from build123d import *

# Parameters (mm, degrees)
SKETCH1_W               = 2.3
SKETCH1_H               = 5.5
SKETCH1_R               = 2.25
BOSS_EXTRUDE1_DEPTH     = 15
CUT_EXTRUDE1_DEPTH      = 33.128647653
CUT_EXTRUDE1_DEPTH_BACK = 33.128647653
SKETCH2_R               = 1.75
FILLET2_R               = 1.5
SKETCH4_R               = 5
CUT_EXTRUDE2_DEPTH      = 10


with BuildPart() as part:
    # Sketch1 → Boss-Extrude1 (new body)
    with BuildSketch(Plane(origin=(0, 0, 0), x_dir=(1, 0, 0), z_dir=(0, 1, 0))):
        with BuildLine():
            Line((15.13, 6.5), (-15.13, 6.5))
            ThreePointArc((-15.13, 6.5), (-18.573610024, 5.073610024), (-20, 1.63))
            Line((-20, 1.63), (-20, -1.63))
            ThreePointArc((-20, -1.63), (-18.573610024, -5.073610024), (-15.13, -6.5))
            Line((-15.13, -6.5), (-6.5, -6.5))
            ThreePointArc((-6.5, -6.5), (-5.439339828, -6.939339828), (-5, -8))
            Line((-5, -8), (-5, -12))
            ThreePointArc((-5, -12), (-4.560660172, -13.060660172), (-3.5, -13.5))
            Line((-3.5, -13.5), (-1, -13.5))
            Line((-1, -13.5), (-1, -3.97617907))
            ThreePointArc((-1, -3.97617907), (-2.520912533, 3.233419243), (4.1, 0))
            ThreePointArc((4.1, 0), (3.233419243, -2.520912533), (1, -3.97617907))
            Line((1, -3.97617907), (1, -13.5))
            Line((1, -13.5), (5.587465673, -13.5))
            Line((5.587465673, -13.5), (7.087465673, -13.5))
            ThreePointArc((7.087465673, -13.5), (8.148125845, -13.060660172), (8.587465673, -12))
            Line((8.587465673, -12), (8.587465673, -8))
            ThreePointArc((8.587465673, -8), (9.026805501, -6.939339828), (10.087465673, -6.5))
            Line((10.087465673, -6.5), (15.13, -6.5))
            ThreePointArc((15.13, -6.5), (18.573610024, -5.073610024), (20, -1.63))
            Line((20, -1.63), (20, 1.63))
            ThreePointArc((20, 1.63), (18.573610024, 5.073610024), (15.13, 6.5))
        make_face()
        with Locations((5, -10)):
            Rectangle(SKETCH1_W, SKETCH1_H, mode=Mode.SUBTRACT)
        with Locations(Location((-13, 0, 0), (0, 0, 270))):
            Circle(SKETCH1_R, mode=Mode.SUBTRACT)
        with Locations(Location((13, 0, 0), (0, 0, 270))):
            Circle(SKETCH1_R, mode=Mode.SUBTRACT)
    extrude(amount=BOSS_EXTRUDE1_DEPTH)

    # Sketch2 → Cut-Extrude1 (cut, two sides: drawn at the far end of the back side and taken through both)
    with BuildSketch(Plane(origin=(5, 0, 0), x_dir=(0, 0, -1), z_dir=(1, 0, 0)).offset(-CUT_EXTRUDE1_DEPTH_BACK)):
        with Locations((-10, 7.5)):
            Circle(SKETCH2_R)
    extrude(amount=CUT_EXTRUDE1_DEPTH + CUT_EXTRUDE1_DEPTH_BACK, mode=Mode.SUBTRACT)

    # Fillet2
    # the kernel refuses this fillet: 1.5 mm, written as the material it takes off along each edge
    with BuildSketch(Plane(origin=(7.087465673, 15, 13.5), x_dir=(0, 0, -1), z_dir=(-1, 0, 0))) as fillet2_piece_1:
        with BuildLine():
            CenterArc((FILLET2_R, FILLET2_R), FILLET2_R, 180, 90)
            Line((0, FILLET2_R), (0, 0))
            Line((0, 0), (FILLET2_R, 0))
        make_face()
    extrude(amount=9.837465673, mode=Mode.SUBTRACT)
    with BuildSketch(Plane(origin=(10.087465673, 15, 6.5), x_dir=(0, 0, -1), z_dir=(1, 0, 0))) as fillet2_piece_2:
        with BuildLine():
            CenterArc((FILLET2_R, -FILLET2_R), FILLET2_R, 90, 90)
            Line((0, -FILLET2_R), (0, 0))
            Line((0, 0), (FILLET2_R, 0))
        make_face()
    extrude(amount=5.042534327, mode=Mode.SUBTRACT)
    with BuildSketch(Plane(origin=(15.13, 15, 1.63), x_dir=(0, 0, 1), z_dir=(-1, 0, 0))) as fillet2_piece_3:
        with BuildLine():
            CenterArc((4.87 - FILLET2_R, -FILLET2_R), FILLET2_R, 0, 90)
            Line((4.87, -FILLET2_R), (4.87, 0))
            Line((4.87, 0), (4.87 - FILLET2_R, 0))
        make_face()
    revolve(axis=Axis((15.13, 15, 1.63), (0, 1, 0)), revolution_arc=90, mode=Mode.SUBTRACT)
    with BuildSketch(Plane(origin=(20, 15, 1.63), x_dir=(-1, 0, 0), z_dir=(0, 0, -1)), Plane(origin=(-20, 15, -1.63), x_dir=(1, 0, 0), z_dir=(0, 0, 1))) as fillet2_piece_4:
        with BuildLine():
            CenterArc((FILLET2_R, -FILLET2_R), FILLET2_R, 90, 90)
            Line((0, -FILLET2_R), (0, 0))
            Line((0, 0), (FILLET2_R, 0))
        make_face()
    extrude(amount=3.26, mode=Mode.SUBTRACT)
    with BuildSketch(Plane(origin=(15.13, 15, -1.63), x_dir=(1, 0, 0), z_dir=(0, 0, 1))) as fillet2_piece_5:
        with BuildLine():
            CenterArc((4.87 - FILLET2_R, -FILLET2_R), FILLET2_R, 0, 90)
            Line((4.87, -FILLET2_R), (4.87, 0))
            Line((4.87, 0), (4.87 - FILLET2_R, 0))
        make_face()
    revolve(axis=Axis((15.13, 15, -1.63), (0, 1, 0)), revolution_arc=90, mode=Mode.SUBTRACT)
    with BuildSketch(Plane(origin=(15.13, 15, -6.5), x_dir=(0, 0, 1), z_dir=(-1, 0, 0))) as fillet2_piece_6:
        with BuildLine():
            CenterArc((FILLET2_R, -FILLET2_R), FILLET2_R, 90, 90)
            Line((0, -FILLET2_R), (0, 0))
            Line((0, 0), (FILLET2_R, 0))
        make_face()
    extrude(amount=30.26, mode=Mode.SUBTRACT)
    with BuildSketch(Plane(origin=(-15.13, 15, -1.63), x_dir=(0, 0, -1), z_dir=(1, 0, 0))) as fillet2_piece_7:
        with BuildLine():
            CenterArc((4.87 - FILLET2_R, -FILLET2_R), FILLET2_R, 0, 90)
            Line((4.87, -FILLET2_R), (4.87, 0))
            Line((4.87, 0), (4.87 - FILLET2_R, 0))
        make_face()
    revolve(axis=Axis((-15.13, 15, -1.63), (0, 1, 0)), revolution_arc=90, mode=Mode.SUBTRACT)
    with BuildSketch(Plane(origin=(-3.5, 15, 13.5), x_dir=(0, 0, -1), z_dir=(1, 0, 0))) as fillet2_piece_8:
        with BuildLine():
            CenterArc((FILLET2_R, -FILLET2_R), FILLET2_R, 90, 90)
            Line((0, -FILLET2_R), (0, 0))
            Line((0, 0), (FILLET2_R, 0))
        make_face()
    extrude(amount=6.25, mode=Mode.SUBTRACT)
    with BuildSketch(Plane(origin=(-3.5, 15, 12), x_dir=(-1, 0, 0), z_dir=(0, 0, -1))) as fillet2_piece_9:
        with BuildLine():
            CenterArc((1.5 - FILLET2_R, -FILLET2_R), FILLET2_R, 0, 90)
            Line((1.5, -FILLET2_R), (1.5, 0))
            Line((1.5, 0), (1.5 - FILLET2_R, 0))
        make_face()
    revolve(axis=Axis((-3.5, 15, 12), (0, 1, 0)), revolution_arc=90, mode=Mode.SUBTRACT)
    with BuildSketch(Plane(origin=(-5, 15, 8), x_dir=(1, 0, 0), z_dir=(0, 0, 1)), Plane(origin=(8.587465673, 15, 12), x_dir=(-1, 0, 0), z_dir=(0, 0, -1))) as fillet2_piece_10:
        with BuildLine():
            CenterArc((FILLET2_R, -FILLET2_R), FILLET2_R, 90, 90)
            Line((0, -FILLET2_R), (0, 0))
            Line((0, 0), (FILLET2_R, 0))
        make_face()
    extrude(amount=4, mode=Mode.SUBTRACT)
    with BuildSketch(Plane(origin=(-6.5, 15, 8), x_dir=(0, 0, -1), z_dir=(-1, 0, 0))) as fillet2_piece_11:
        with BuildLine():
            CenterArc((1.5 + FILLET2_R, FILLET2_R), FILLET2_R, 180, 90)
            Line((1.5, FILLET2_R), (1.5, 0))
            Line((1.5, 0), (1.5 + FILLET2_R, 0))
        make_face()
    revolve(axis=Axis((-6.5, 15, 8), (0, -1, 0)), revolution_arc=90, mode=Mode.SUBTRACT)
    with BuildSketch(Plane(origin=(-15.13, 15, 1.63), x_dir=(-1, 0, 0), z_dir=(0, 0, -1))) as fillet2_piece_12:
        with BuildLine():
            CenterArc((4.87 - FILLET2_R, -FILLET2_R), FILLET2_R, 0, 90)
            Line((4.87, -FILLET2_R), (4.87, 0))
            Line((4.87, 0), (4.87 - FILLET2_R, 0))
        make_face()
    revolve(axis=Axis((-15.13, 15, 1.63), (0, 1, 0)), revolution_arc=90, mode=Mode.SUBTRACT)
    with BuildSketch(Plane(origin=(-15.13, 15, 6.5), x_dir=(0, 0, -1), z_dir=(1, 0, 0))) as fillet2_piece_13:
        with BuildLine():
            CenterArc((FILLET2_R, -FILLET2_R), FILLET2_R, 90, 90)
            Line((0, -FILLET2_R), (0, 0))
            Line((0, 0), (FILLET2_R, 0))
        make_face()
    extrude(amount=8.63, mode=Mode.SUBTRACT)
    with BuildSketch(Plane(origin=(7.087465673, 15, 12), x_dir=(0, 0, 1), z_dir=(-1, 0, 0))) as fillet2_piece_14:
        with BuildLine():
            CenterArc((1.5 - FILLET2_R, -FILLET2_R), FILLET2_R, 0, 90)
            Line((1.5, -FILLET2_R), (1.5, 0))
            Line((1.5, 0), (1.5 - FILLET2_R, 0))
        make_face()
    revolve(axis=Axis((7.087465673, 15, 12), (0, 1, 0)), revolution_arc=90, mode=Mode.SUBTRACT)
    with BuildSketch(Plane(origin=(10.087465673, 15, 8), x_dir=(-1, 0, 0), z_dir=(0, 0, 1))) as fillet2_piece_15:
        with BuildLine():
            CenterArc((1.5 + FILLET2_R, FILLET2_R), FILLET2_R, 180, 90)
            Line((1.5, FILLET2_R), (1.5, 0))
            Line((1.5, 0), (1.5 + FILLET2_R, 0))
        make_face()
    revolve(axis=Axis((10.087465673, 15, 8), (0, -1, 0)), revolution_arc=90, mode=Mode.SUBTRACT)

    # Sketch4 → Cut-Extrude2 (cut)
    with BuildSketch(Plane(origin=(0, 15, 0), x_dir=(1, 0, 0), z_dir=(0, 1, 0))):
        with Locations(Location((-13, 0, 0), (0, 0, 270))):
            Circle(SKETCH4_R)
        with Locations(Location((13, 0, 0), (0, 0, 270))):
            Circle(SKETCH4_R)
    extrude(amount=-CUT_EXTRUDE2_DEPTH, mode=Mode.SUBTRACT)


solid = part.part
Read the model definition and answer for the solid it produces. Units are mm, in the model's axes. A direction names the side the tool comes from. Give positions to 0.01 mm unless a question says otherwise; leave off trailing zeros. Write each loop counter-clockwise with the first axis right and the second up, starting at its lowest first coordinate (ties: lowest second). Pieces come first, ordered by that corner, then holes. Notation, with made-up numbers: (55.5, 17) - (77.5, 17) arc R23 cw to (77.5, 53) - close; hole circle Ø1 at (-34, 80). An arc over 180 degrees is marked (long way). Use CSV: the item, a comma, the result in double quotes. Start each with the question number.
(1) Find section D-D (y = 7.5). Count the separate pieces of the cut face and the enclosed holes in it, plus the area to 3 significant figures.
(2) Consider line 1 along X through (y, z) = (3.4, 0); line 2 along X through (y, z) = (5, 10.25); line 3 along X through (y, z) = (11.25, 0.5). Determine where each line is inside the solid, lowest interval first.
(3) Find section A-A (z = 10). Give the vertices of the cut face in (x, y), plus the area to 3 significant figures.
(4) Given P1, Ø5.5, axis at y = 7.5, z = 10, coming from the -X side; P2, Ø2, axis at y = 9.5, z = 10.5, coming from the +X side; P3, Ø1.6, axis at y = 4.5, z = 9, coming from the -X side, each flat-ended and moving along its own axis, determine where each tip first touches the part or whether it passes through.
(5) Find section C-C (x = -3). Give the vertices of the cut face in (y, z).
(6) Find section B-B (y = 2). Give the vertices of the cut face in (x, z).
(7) For faces 1 (the flat face through (6.15, 7, 8)), 2 (the cylindrical face through (17.957, 10.07, -0.651)), 3 (the flat face through (-5, 5, 10)), 4 (the flat face through (8.587, 5, 10)), determine the directions among +Z, -Z, +X, -X, +Y, -Y from which every point of the face is accessible in a straight line to the end or side of a thin tool.
(8) Determine the mould class of faces 5 (the cylindrical face through (15.23, 2.46, -0.29)), 6 (the flat face through (20, 7, 0)), 7 (the cylindrical face through (-3.028, 6.83, 8.383)), 8 (the flat face through (4, 7, 13.5)) for opening direction Z: +Z half, -Z half, draft (parallel to the pull), parting line (faces both ways), or undercut.
Findings below:
1,separate pieces,"3"
1,enclosed holes,"2"
1,area,"321 mm2"
2,line 1,"-20 to -15.25, -10.75 to -4.1, 4.1 to 10.75, 15.25 to 20"
2,line 2,"-5 to -1, 1 to 3.85, 6.15 to 8.59"
2,line 3,"-20 to -17.97, -8.03 to -4.07, 4.07 to 8.03, 17.97 to 20"
3,outline,"(-5, 0) - (-1, 0) - (-1, 5.75) - (-5, 5.75) - close; (-5, 9.25) - (-1, 9.25) - (-1, 15) - (-3.5, 15) arc R1.5 ccw to (-5, 13.5) - close; (1, 0) - (3.85, 0) - (3.85, 5.75) - (1, 5.75) - close; (1, 9.25) - (3.85, 9.25) - (3.85, 15) - (1, 15) - close; (6.15, 0) - (8.59, 0) - (8.59, 5.75) - (6.15, 5.75) - close; (6.15, 9.25) - (8.59, 9.25) - (8.59, 13.5) arc R1.5 ccw to (7.09, 15) - (6.15, 15) - close"
3,area,"106 mm2"
4,P1,"x = -5.2"
4,P2,"x = 8.59"
4,P3,"x = -5"
5,outline,"(0, -6.5) - (13.5, -6.5) arc R1.5 ccw to (15, -5) - (15, -2.79) - (0, -2.79) - close; (0, 2.79) - (15, 2.79) - (15, 12) arc R1.5 ccw to (13.5, 13.5) - (0, 13.5) - close; hole circle Ø3.5 at (7.5, 10)"
6,outline,"(-20, -1.63) arc R4.87 ccw to (-15.13, -6.5) - (15.13, -6.5) arc R4.87 ccw to (20, -1.63) - (20, 1.63) arc R4.87 ccw to (15.13, 6.5) - (10.09, 6.5) arc R1.5 cw to (8.59, 8) - (8.59, 12) arc R1.5 ccw to (7.09, 13.5) - (1, 13.5) - (1, 3.98) arc R4.1 cw (long way) to (-1, 3.98) - (-1, 13.5) - (-3.5, 13.5) arc R1.5 ccw to (-5, 12) - (-5, 8) arc R1.5 cw to (-6.5, 6.5) - (-15.13, 6.5) arc R4.87 ccw to (-20, 1.63) - close; hole circle Ø4.5 at (-13, 0); hole (3.85, 7.25) - (6.15, 7.25) - (6.15, 12.75) - (3.85, 12.75) - close; hole circle Ø4.5 at (13, 0)"
7,face 1,"+Y, -Y"
7,face 2,"+Y"
7,face 3,"+Z, -X, +Y, -Y"
7,face 4,"+Z, +X, +Y, -Y"
8,face 5,"undercut"
8,face 6,"draft"
8,face 7,"undercut"
8,face 8,"+Z half"
